Read the model definition and answer for the solid it produces. Units are mm, in the model's axes. A direction names the side the tool comes from. Round coordinates to 2 decimals unless told otherwise and drop trailing zeros. Order: outer loops, then holes, each group sorted by start corner. A loop starts at its lowest first (then second) coordinate and runs counter-clockwise, first axis right, second up. Notation, with made-up numbers: (-23.75, 49.25) -> (-18.75, 49.25) arc R22 ccw to (-18.75, 56.25) -> close; hole circle Ø1 at (88, 78). An arc over 180 degrees is marked (long way). Answer as a JSON object with one key per item and string values. Group by question number.
Item 1: The mould has two halves that part along Z. Classify faces 1 (the flat face through (11.5, 4, 0)), 2 (the cylindrical face through (9.38, 7.81, -1.73)), 3 (the flat face through (14, 3, 3)): pulls with the +Z half, pulls with the -Z half, needs draft (parallel to the pull), parting line crosses it, or undercut.
Item 2: Section A-A, the plane y = 0 is taken. Write down the section's boundary in (x, z).
Item 3: For faces 4 (the cylindrical face through (12.74, 1.978, -2.579)), 5 (the cylindrical face through (8.28, 3.13, -4.09)), determine the directions among +Z, -Z, +X, -X, +Y, -Y from which every point of the face is accessible in a straight line to the end or side of a thin tool.
Item 4: Consider probe 1 along Y at (x, z) = (7.5, 0); probe 2 along Y at (x, z) = (13, 0); probe 3 along Z at (x, y) = (11, -3.75). Determine where each line is inside the solid, lowest interval first. Write a range as from..to.
Item 5: Given P1, Ø1.5, axis at x = 7.5, y = -6.5, coming from the +Z side; P2, Ø2, axis at x = 12.5, y = 6, coming from the +Z side (3 decimals); P3, Ø1.5, axis at x = 6.5, z = -1.5, coming from the -Y side, each flat-ended and moving along its own axis, determine where each tip first touches the part or whether it passes through.
Item 6: Section C-C, the plane x = 12.25 is taken. Write down the section's boundary in (y, z), plus the area to 3 significant figures.
Item 7: Section D-D, the plane x = 7 is taken. Write down the section's boundary in (y, z).
from build123d import *

# Parameters (mm, degrees)
CUT_EXTRUDE1_DEPTH      = 19
CUT_EXTRUDE1_DEPTH_BACK = 19
SKETCH2_R               = 3.25
FILLET1_R               = 0.5


with BuildPart() as part:
    # Sketch1 → Revolve1 (revolve)
    with BuildSketch(Plane.XY, mode=Mode.PRIVATE) as revolve1_sk:
        Polygon((11.5, 5.15), (4.65, 5.15), (4.65, 8), (14, 8), (14, 0), (11.5, 0), align=None)
    revolve(revolve1_sk.sketch.rotate(Axis((-1.174323487, 0, 0), (1, 0, 0)), 90), axis=Axis((-1.174323487, 0, 0), (1, 0, 0)))

    # Sketch2 → Cut-Extrude1 (cut, two sides: drawn at the far end of the back side and taken through both)
    with BuildSketch(Plane(origin=(0, 0, 0), x_dir=(0, 0, -1), z_dir=(1, 0, 0)).offset(-CUT_EXTRUDE1_DEPTH_BACK)):
        with Locations(Location((0, 0, 0), (0, 0, 180))):
            Circle(SKETCH2_R)
    extrude(amount=CUT_EXTRUDE1_DEPTH + CUT_EXTRUDE1_DEPTH_BACK, mode=Mode.SUBTRACT)

    # Fillet1
    fillet1_edges = [part.edges().sort_by_distance(p)[0] for p in [
        (11.5, 0, -3.25),
        (14, 0, -3.25),
        (4.65, 0, -5.15),
        (4.65, 0, -8),
        (14, 0, -8),
    ]]
    fillet(fillet1_edges, radius=FILLET1_R)


solid = part.part
Values found:
{
 "1": {"face 1": "undercut", "face 2": "parting line crosses it", "face 3": "needs draft"},
 "2": {"outline": "(4.65, -7.5) arc R0.5 ccw to (5.15, -8) -> (13.5, -8) arc R0.5 ccw to (14, -7.5) -> (14, -3.75) arc R0.5 ccw to (13.5, -3.25) -> (12, -3.25) arc R0.5 ccw to (11.5, -3.75) -> (11.5, -5.15) -> (5.15, -5.15) arc R0.5 ccw to (4.65, -5.65) -> close; (4.65, 5.65) arc R0.5 ccw to (5.15, 5.15) -> (11.5, 5.15) -> (11.5, 3.75) arc R0.5 ccw to (12, 3.25) -> (13.5, 3.25) arc R0.5 ccw to (14, 3.75) -> (14, 7.5) arc R0.5 ccw to (13.5, 8) -> (5.15, 8) arc R0.5 ccw to (4.65, 7.5) -> close"},
 "3": {"face 4": "+X, -X", "face 5": "-X"},
 "4": {"probe 1": "-8..-5.15, 5.15..8", "probe 2": "-8..-3.25, 3.25..8", "probe 3": "-7.07..-3.53, 3.53..7.07"},
 "5": {"P1": "z = 5.56", "P2": "z = 6.245", "P3": "y = -7.96"},
 "6": {"outline": "circle Ø16 at (0, 0); hole circle Ø6.5 at (0, 0)", "area": "168 mm2"},
 "7": {"outline": "circle Ø16 at (0, 0); hole circle Ø10.3 at (0, 0)"}
}
